Study the drawing (mm; zero at the part's minimum x, y, z) and answer. A direction names the side the tool comes from. Round coordinates to 2 decimals unless told otherwise and drop trailing zeros. Loops run counter-clockwise (first coordinate to the right, second up) from the corner with the lowest first, then second, coordinate; pieces in that order, holes last. Notation, with made-up numbers: (57.5, 53) -> (102.5, 53) arc R11 ccw to (102.5, 62) -> close; hole circle Ø7 at (76.25, -28.5). An arc over 180 degrees is marked (long way). Use one line per item in the form item = value.
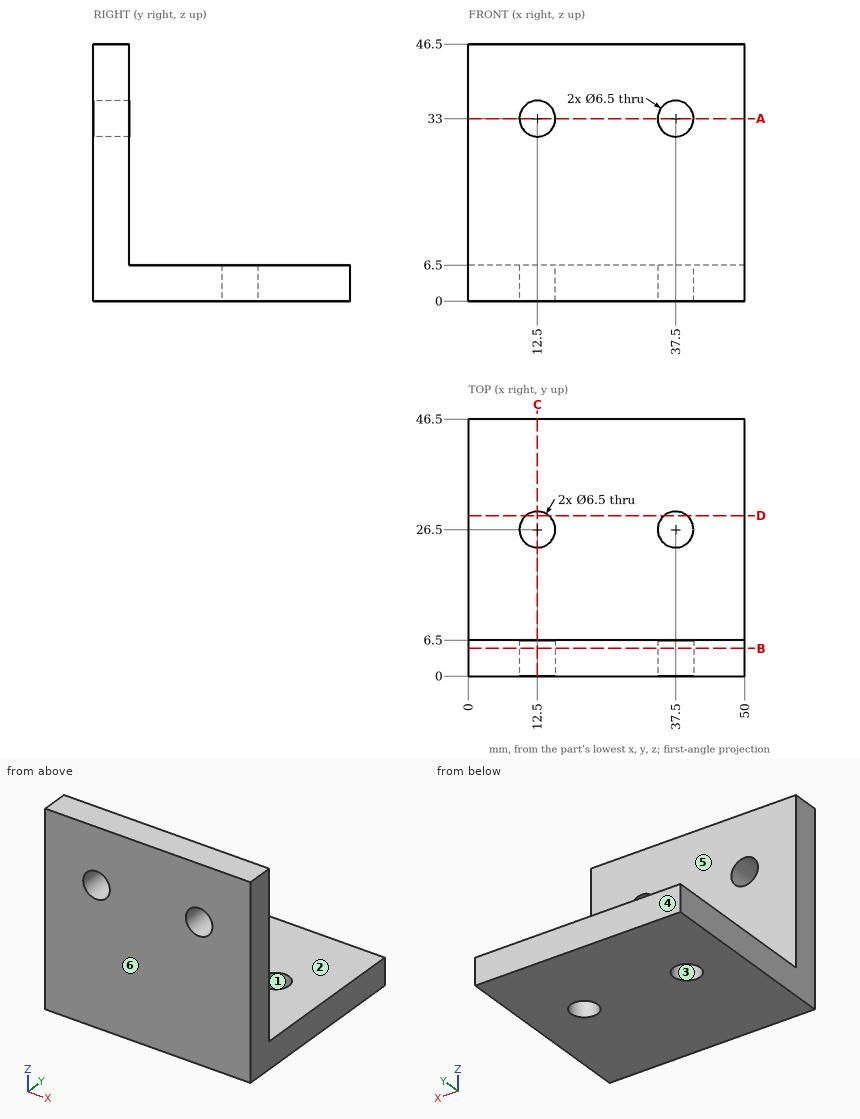
(1) Consider L1, parallel to X at y = 4, z = 33; L2, parallel to Z at x = 12.5, y = 4; L3, parallel to Z at x = 23.5, y = 13.5. Determine where each line is inside the solid, lowest interval first.
Completed:
L1 = 0 to 9.25, 15.75 to 34.25, 40.75 to 50
L2 = 0 to 29.75, 36.25 to 46.5
L3 = 0 to 6.5
(2) Find section A-A, the plane z = 33. Write down the section's boundary in (x, y), then the cut area to 4 significant figures.
Completed:
outline = (0, 0) -> (9.25, 0) -> (9.25, 6.5) -> (0, 6.5) -> close; (15.75, 0) -> (34.25, 0) -> (34.25, 6.5) -> (15.75, 6.5) -> close; (40.75, 0) -> (50, 0) -> (50, 6.5) -> (40.75, 6.5) -> close
area = 240.5 mm2
(3) For a pull along Y with two mould halves and no side action, classify the marked faces 1, 2, 3 and 4 as +Y half, -Y half, draft (parallel to the pull), parting line (faces both ways), or undercut.
Completed:
face_1 = undercut
face_2 = draft
face_3 = undercut
face_4 = +Y half
(4) Find section B-B, the plane y = 5. Write down the section's boundary in (x, z), then the cut area to 3 significant figures.
Completed:
outline = (0, 0) -> (50, 0) -> (50, 46.5) -> (0, 46.5) -> close; hole circle Ø6.5 at (12.5, 33); hole circle Ø6.5 at (37.5, 33)
area = 2,260 mm2
(5) Find section D-D, the plane y = 29. Write down the section's boundary in (x, z).
Completed:
outline = (0, 0) -> (10.42, 0) -> (10.42, 6.5) -> (0, 6.5) -> close; (14.58, 0) -> (35.42, 0) -> (35.42, 6.5) -> (14.58, 6.5) -> close; (39.58, 0) -> (50, 0) -> (50, 6.5) -> (39.58, 6.5) -> close
(6) For the marked faces 5 and 6, determine the directions among +Z, -Z, +X, -X, +Y, -Y from which every point of the face is accessible in a straight line to the end or side of a thin tool.
Completed:
face_5 = +Z, +X, -X, +Y
face_6 = +Z, -Z, +X, -X, -Y
(7) Given P1, Ø12, axis at x = 33, y = 21, coming from the +Z side; P2, Ø4, axis at x = 14.5, z = 31.5, coming from the +Y side, each flat-ended and moving along its own axis, determine where each tip first touches the part or whether it passes through.
Completed:
P1 = 6.5
P2 = 6.5
(8) Find section C-C, the plane x = 12.5. Write down the section's boundary in (y, z), then the cut area to 3 significant figures.
Completed:
outline = (0, 0) -> (23.25, 0) -> (23.25, 6.5) -> (6.5, 6.5) -> (6.5, 29.75) -> (0, 29.75) -> close; (0, 36.25) -> (6.5, 36.25) -> (6.5, 46.5) -> (0, 46.5) -> close; (29.75, 0) -> (46.5, 0) -> (46.5, 6.5) -> (29.75, 6.5) -> close
area = 478 mm2
